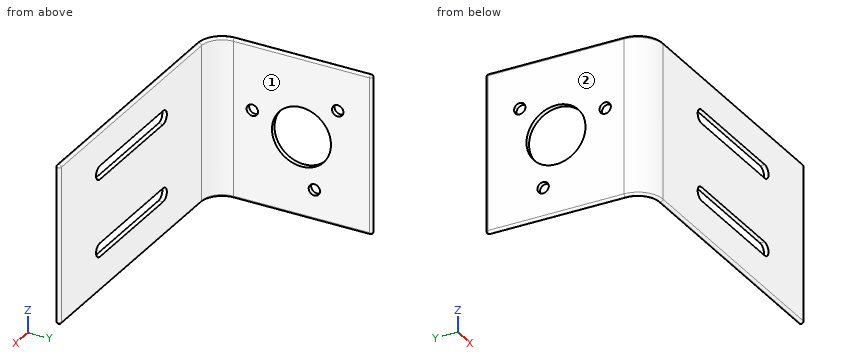
from build123d import *

# Parameters (mm, degrees)
BOSS_EXTRUDE1_DEPTH   = 35
CUT_EXTRUDE1_REACH    = 80.316
SKETCH3_R             = 6.5
FILLET1_R             = 0.5
CUT_EXTRUDE3_DEPTH    = 35
F_2_5MM_DOWEL_HOLE1_D = 2.5


with BuildPart() as part:
    # Sketch1 → Boss-Extrude1 (new body)
    with BuildSketch(Plane.XY):
        with BuildLine():
            Line((0, 0.5), (-55.4, 0.5))
            ThreePointArc((-55.4, 0.5), (-58.581980515, 1.818019485), (-59.9, 5))
            Line((-59.9, 5), (-59.9, 35))
            ThreePointArc((-59.9, 35), (-60.4, 35.5), (-60.9, 35))
            Line((-60.9, 35), (-60.9, 5))
            ThreePointArc((-60.9, 5), (-59.289087297, 1.110912703), (-55.4, -0.5))
            Line((-55.4, -0.5), (0, -0.5))
            ThreePointArc((0, -0.5), (0.5, 0), (0, 0.5))
        make_face()
    extrude(amount=BOSS_EXTRUDE1_DEPTH)

    # Sketch3 → Cut-Extrude1 (cut, up to next)
    with BuildSketch(Plane(origin=(-59.9, 0, 0), x_dir=(0, 0, -1), z_dir=(1, 0, 0)), mode=Mode.PRIVATE) as cut_extrude1_sk1:
        with Locations(Location((-17.5, 20, 0), (0, 0, 90))):
            Circle(SKETCH3_R)
    cut_extrude1_tool1 = extrude(cut_extrude1_sk1.sketch, amount=-CUT_EXTRUDE1_REACH, mode=Mode.PRIVATE) & part.part
    add(cut_extrude1_tool1.solids().sort_by_distance((-59.9, 20, 17.5))[0], mode=Mode.SUBTRACT)

    # Fillet1
    fillet1_edges = [part.edges().sort_by_distance(p)[0] for p in [
        (-60.9, 20, 0),
        (-60.4, 35.5, 0),
        (-59.9, 20, 0),
        (-58.581980515, 1.818019485, 0),
        (-60.4, 35.5, 35),
        (-60.9, 20, 35),
        (-59.289087297, 1.110912703, 35),
        (-27.7, -0.5, 35),
        (0.5, 0, 35),
        (-27.7, 0.5, 35),
        (-58.581980515, 1.818019485, 35),
        (-27.7, 0.5, 0),
        (-59.9, 20, 35),
        (0.5, 0, 0),
        (-27.7, -0.5, 0),
        (-59.289087297, 1.110912703, 0),
    ]]
    fillet(fillet1_edges, radius=FILLET1_R - 0.0001)  # a hair under: the kernel refuses the full size

    # Sketch6 → Cut-Extrude3 (cut)
    with BuildSketch(Plane(origin=(0, 0.5, 0), x_dir=(1, 0, 0), z_dir=(0, 1, 0))):
        with BuildLine():
            Line((-40.2, -7.5), (-15.2, -7.5))
            ThreePointArc((-15.2, -7.5), (-13.7, -9), (-15.2, -10.5))
            Line((-15.2, -10.5), (-40.2, -10.5))
            ThreePointArc((-40.2, -10.5), (-41.7, -9), (-40.2, -7.5))
        make_face()
        with BuildLine():
            Line((-40.2, -27.5), (-15.2, -27.5))
            ThreePointArc((-15.2, -27.5), (-13.7, -26), (-15.2, -24.5))
            Line((-15.2, -24.5), (-40.2, -24.5))
            ThreePointArc((-40.2, -24.5), (-41.7, -26), (-40.2, -27.5))
        make_face()
    extrude(amount=-CUT_EXTRUDE3_DEPTH, mode=Mode.SUBTRACT)

    # Ø2.5mm Dowel Hole1 (through all)
    with Locations(Plane(origin=(-59.9, 27.981374836, 25.385813574), x_dir=(0, 1, 0), z_dir=(1, 0, 0))):
        with Locations((0, 0), (-18.801377139, -4.916646995), (-5.14274737, -18.740793726)):
            Hole(F_2_5MM_DOWEL_HOLE1_D / 2)


solid = part.part
CAD build for the part. Positions are in the model's coordinates, mm. Face numbers are marked on the shaded views. A direction names the side the tool comes from. Round coordinates to 2 decimals unless told otherwise and drop trailing zeros. Loops run counter-clockwise (first coordinate to the right, second up) from the corner with the lowest first, then second, coordinate; pieces in that order, holes last. Notation, with made-up numbers: M 10,53.5 L 56,53.5 A17 ccw 56,69.5 Z; hole C 23,55.5 d3. An arc over 180 degrees is marked long. One line per question, with ' | ' between items. Start each with the question number.
Item 1: Wall check: line 1 (Y direction, x = -8, z = 25); line 2 (X direction, y = 33.5, z = 7.5); line 3 (Z direction, x = -60.15, y = 20). Give the ranges that are in metal, low to high.
Item 2: Pin check, flat tip, straight feed: pin 1 Ø2 at (y, z) = (16.5, 24.5) entering from +X. Stop position of the tip, or through.
Item 3: Which spindle directions (+Z, -Z, +X, -X, +Y, -Y) get a long thin tool onto all of the face, cutting with end or side? Do the marked faces 1 and 2. Say none if no direction does.
Item 4: Cut at B-B, the plane x = -39.5. State how many separate pieces and enclosed holes the cut face has, plus the area to 3 significant figures.
Item 5: Cut at A-A, the plane z = 9. Write the cut outline in (x, y), plus the area to 3 significant figures.
Responses:
1) line 1: y = -0.5 to 0.5 | line 2: x = -60.9 to -59.9 | line 3: z = 0.07 to 11, 24 to 34.93
2) pin 1: stops at x = -59.9
3) face 1: +Z, -Z, +X, +Y | face 2: +Z, -Z, -X, +Y, -Y
4) separate pieces: 3 | enclosed holes: 0 | area: 28.8 mm²
5) outline: M -60.9,5 A5.5 ccw -55.4,-0.5 L -41.7,-0.5 L -41.7,0.5 L -55.4,0.5 A4.5 cw -59.9,5 L -59.9,35 A0.5 ccw -60.9,35 Z; M -13.7,-0.5 L 0,-0.5 A0.5 ccw 0,0.5 L -13.7,0.5 Z | area: 66.0 mm²
